```python
from build123d import *

# Parameters (mm, degrees)
F0_R     = 2
F3_DEPTH = 32.004
F0_R_2   = 4
F0_R_3   = 0.5
F4_DEPTH = 5
F5_DEPTH = 5.5
F6_DEPTH = 7
F7_R     = 3
F7_R_2   = 2
F8_DEPTH = 8
F7_R_3   = 17.816411
F7_R_4   = 9.257541
F9_DEPTH = 12.7


with BuildPart() as f2:
    # F1 (on Right) → F2 (revolve)
    with BuildSketch(Plane.YZ):
        with BuildLine():
            Line((-3, 0), (0, 0))
            Line((0, 0), (0, 19.5))
            Line((0, 19.5), (-16, 19.5))
            ThreePointArc((-16, 19.5), (-17, 14), (-16, 8.5))
            Line((-16, 8.5), (-3, 8.5))
            Line((-3, 8.5), (-3, 0))
        make_face()
    revolve(axis=Axis((0, -1.5, 0), (0, 1, 0)))

    # F0 (on Front) → F3 (cut)
    with BuildSketch(Plane.XZ):
        with Locations((0, 6.25)):
            Circle(F0_R)
        with Locations((-4.419418, 4.419418)):
            Circle(F0_R)
        with Locations((-6.25, 0)):
            Circle(F0_R)
        with Locations((-4.419418, -4.419418)):
            Circle(F0_R)
        with Locations((0, -6.25)):
            Circle(F0_R)
        with Locations((4.419418, -4.419418)):
            Circle(F0_R)
        with Locations((6.25, 0)):
            Circle(F0_R)
        with Locations((4.419418, 4.419418)):
            Circle(F0_R)
    extrude(amount=F3_DEPTH, mode=Mode.SUBTRACT)

    # F0 (on Front) → F4 (join)
    with BuildSketch(Plane.XZ):
        Circle(F0_R_2)
        with Locations((-0.927052, -2.853171)):
            Circle(F0_R_3, mode=Mode.SUBTRACT)
        with Locations((-2.427053, -1.763357)):
            Circle(F0_R_3, mode=Mode.SUBTRACT)
        with Locations((0.927052, -2.853171)):
            Circle(F0_R_3, mode=Mode.SUBTRACT)
        with Locations((2.427053, -1.763357)):
            Circle(F0_R_3, mode=Mode.SUBTRACT)
        with Locations((-3.000002, 0)):
            Circle(F0_R_3, mode=Mode.SUBTRACT)
        with Locations((-2.427053, 1.763357)):
            Circle(F0_R_3, mode=Mode.SUBTRACT)
        with Locations((-0.927052, 2.853171)):
            Circle(F0_R_3, mode=Mode.SUBTRACT)
        Circle(F0_R, mode=Mode.SUBTRACT)
        with Locations((2.427053, 1.763357)):
            Circle(F0_R_3, mode=Mode.SUBTRACT)
        with Locations((3.000002, 0)):
            Circle(F0_R_3, mode=Mode.SUBTRACT)
        with Locations((0.927052, 2.853171)):
            Circle(F0_R_3, mode=Mode.SUBTRACT)
    extrude(amount=F4_DEPTH)

    # F0 (on Front) → F5 (join)
    with BuildSketch(Plane.XZ):
        with Locations((0.927052, 2.853171)):
            Circle(F0_R_3)
        with Locations((-0.927052, 2.853171)):
            Circle(F0_R_3)
        with Locations((-2.427053, 1.763357)):
            Circle(F0_R_3)
        with Locations((-3.000002, 0)):
            Circle(F0_R_3)
        with Locations((-2.427053, -1.763357)):
            Circle(F0_R_3)
        with Locations((-0.927052, -2.853171)):
            Circle(F0_R_3)
        with Locations((0.927052, -2.853171)):
            Circle(F0_R_3)
        with Locations((2.427053, -1.763357)):
            Circle(F0_R_3)
        with Locations((3.000002, 0)):
            Circle(F0_R_3)
        with Locations((2.427053, 1.763357)):
            Circle(F0_R_3)
    extrude(amount=F5_DEPTH)

    # F0 (on Front) → F6 (join)
    with BuildSketch(Plane.XZ):
        Circle(F0_R)
    extrude(amount=F6_DEPTH)

    # F7 (on face) → F8 (join)
    with BuildSketch(Plane.XZ):
        Circle(F7_R)
        Circle(F7_R_2, mode=Mode.SUBTRACT)
    extrude(amount=-F8_DEPTH)

    # F7 (on face) → F9 (cut)
    with BuildSketch(Plane.XZ):
        Circle(F7_R_3)
        Circle(F7_R_4, mode=Mode.SUBTRACT)
    extrude(amount=F9_DEPTH, mode=Mode.SUBTRACT)


solid = f2.part
```
Can you work these out from the model? Positions are in its coordinate system, mm. A direction names the side the tool comes from. Coordinates: 2 decimals unless noted, no trailing zeros. Write each loop counter-clockwise with the first axis right and the second up, starting at its lowest first coordinate (ties: lowest second). Pieces come first, ordered by that corner, then holes. Notation, with made-up numbers: (3, 65.5) - (9, 65.5) arc R20 ccw to (9, 104.5) - close; hole circle Ø1 at (-32, -17.75). An arc over 180 degrees is marked (long way). Return JSON: item names as keys, results as strings.
Q1. Thinking about a two-plate mould opening in X: for faces 4 (the cylindrical face through (-3, 4, 0)), 5 (the cylindrical face through (-0.26, -1.479, 8.233)), which applies, +X half, -X half, draft (parallel to the pull), parting line (faces both ways), or undercut?
Computed values:
{"face 4": "parting line", "face 5": "undercut"}
Q2. If we section it at A-A (y = -11.5): Please give me the cut outline in (x, z).
Computed values:
{"outline": "circle Ø39 at (0, 0); circle Ø18.52 at (0, 0); hole circle Ø35.63 at (0, 0); hole circle Ø17 at (0, 0)"}
Q3. I'm going to push flat-ended pins straight in: pin 1 Ø2 at (x, z) = (-4, -14) entering from +Y; pin 2 Ø3.5 at (x, z) = (0, 0) entering from +Y; pin 3 Ø1.1 at (x, z) = (-1, -3) entering from -Y; pin 4 Ø9.5 at (x, z) = (1.5, -1) entering from +Y. Where does each tip first touch, or does it pass through?
Computed values:
{"pin 1": "stops at y = -12.7", "pin 2": "stops at y = 0", "pin 3": "stops at y = -5.5", "pin 4": "stops at y = 8"}
Q4. If we section it at C-C (z = 0): Count the separate pieces of the cut face and the enclosed holes in it, then the cut area to 3 significant figures.
Computed values:
{"separate pieces": "3", "enclosed holes": "0", "area": "217 mm2"}
Q5. Please list where these lines run through material, in increasing order: L1, parallel to X at y = -0.25, z = -5.5; L2, parallel to Z at x = -3, y = -4.25; L3, parallel to Y at x = 1.5, z = -4. Write a range as from..to.
Computed values:
{"L1": "x = -18.71..-16.95, -7.45..-6.1, -2.74..-1.85, 1.85..2.74, 6.1..7.45, 16.95..18.71", "L2": "z = -19.27..-17.56, -8.76..-7.95, -2.65..2.65, 7.95..8.76, 17.56..19.27", "L3": "y = -3..0"}
Q6. On a 3-axis mill with a long thin cutter (end or side, diameter ignored), from which of +Z, -Z, +X, -X, +Y, -Y can I reach the whole of each face in a straight line? I mean faces 1 (the flat face through (8, -12.7, -8)), 2 (the cylindrical face through (2.6, -5.2, -0.3)), 3 (the cylindrical face through (-6.417, -1.479, -4.331)). Say none if no direction works.
Computed values:
{"face 1": "+Y", "face 2": "-Y", "face 3": "+Y, -Y"}
Q7. If we section it at B-B (y = 1.75): Please give me the cut outline in (x, z).
Computed values:
{"outline": "circle Ø6 at (0, 0); hole circle Ø4 at (0, 0)"}
